from build123d import *

# Parameters (mm, degrees)
F1_DEPTH = 15
F2_R     = 7.5
F3_DEPTH = 5


with BuildPart() as f1:
    # F0 (on Front) → F1 (new body)
    with BuildSketch(Plane.XZ):
        with BuildLine():
            Line((-20, -25), (20, -25))
            Line((20, -25), (20, -12.536835))
            ThreePointArc((20, -12.536835), (15.923849, -0.018417), (20, 12.5))
            Line((20, 12.5), (20, 25))
            Line((20, 25), (-20, 25))
            Line((-20, 25), (-20, 12.5))
            ThreePointArc((-20, 12.5), (-15.923849, -0.018417), (-20, -12.536835))
            Line((-20, -12.536835), (-20, -25))
        make_face()
    extrude(amount=F1_DEPTH)

    # F2 (on face) → F3 (cut)
    with BuildSketch(Plane(origin=(0, 0, 0), x_dir=(-1, 0, 0), z_dir=(0, 1, 0))):
        Circle(F2_R)
    extrude(amount=-F3_DEPTH, mode=Mode.SUBTRACT)


solid = f1.part
Part model, mm, in its own coordinate system. A direction names the side the tool comes from. Give positions to 0.01 mm unless a question says otherwise; leave off trailing zeros. Loops run counter-clockwise (first coordinate to the right, second up) from the corner with the lowest first, then second, coordinate; pieces in that order, holes last. Notation, with made-up numbers: (-4.5, 54) -> (23.5, 54) arc R15 cw to (23.5, 63) -> close; hole circle Ø1 at (45, 73). An arc over 180 degrees is marked (long way). Write each question's results on one line, items separated by ' | '. Start each with the question number.
Q1. Band-saw the part on B-B on y = -7.75. List the corners of the cut face in (x, z), plus the area to 3 significant figures.
Q2. Which spindle directions (+Z, -Z, +X, -X, +Y, -Y) get a long thin tool onto all of the face, cutting with end or side? Do faces 1 (the face through (7.493, -2.465, 0.33)), 2 (the face through (-20, -7, 19)). Say none if no direction does.
Q3. Band-saw the part on C-C on y = -3. List the corners of the cut face in (x, z).
Q4. Band-saw the part on D-D on z = 11.5. List the corners of the cut face in (x, y).
Q5. Pin check, flat tip, straight feed: P1, Ø3, axis at y = -13.5, z = -6.5, coming from the -X side. Stop position of the tip, or through.
Q6. Band-saw the part on A-A on z = 0. List the corners of the cut face in (x, y).
Q7. Wall check: L1, parallel to Z at x = 0, y = -1.95; L2, parallel to Y at x = 1, z = -3; L3, parallel to X at y = -2.5, z = 6.5. Give the ranges that are in metal, low to high.
Q8. Pull direction Z, two halves, no side cores. Call faces 3 (the face through (0, -5, 0)), 4 (the face through (-20, -7, -19)), 5 (the face through (0, -7, -25)): +Z half, -Z half, draft (parallel to the pull), parting line (faces both ways), or undercut.
Results are:
1) outline: (-20, -25) -> (20, -25) -> (20, -12.54) arc R21.26 cw to (20, 12.5) -> (20, 25) -> (-20, 25) -> (-20, 12.5) arc R21.26 cw to (-20, -12.54) -> close | area: 1,860 mm²
2) face 1: +Y | face 2: +Z, -Z, -X, +Y, -Y
3) outline: (-20, -25) -> (20, -25) -> (20, -12.54) arc R21.26 cw to (20, 12.5) -> (20, 25) -> (-20, 25) -> (-20, 12.5) arc R21.26 cw to (-20, -12.54) -> close; hole circle Ø15 at (0, 0)
4) outline: (-19.31, -15) -> (19.31, -15) -> (19.31, 0) -> (-19.31, 0) -> close
5) P1: stops at x = -17.48
6) outline: (-15.92, -15) -> (15.92, -15) -> (15.92, 0) -> (7.5, 0) -> (7.5, -5) -> (-7.5, -5) -> (-7.5, 0) -> (-15.92, 0) -> close
7) L1: z = -25 to -7.5, 7.5 to 25 | L2: y = -15 to -5 | L3: x = -16.95 to -3.74, 3.74 to 16.95
8) face 3: undercut | face 4: draft | face 5: -Z half
